```python
from build123d import *

# Parameters (mm, degrees)
SKETCH2_W           = 300
SKETCH2_H           = 200
BOSS_EXTRUDE1_DEPTH = 15
SKETCH3_W           = 240
SKETCH3_H           = 140
BOSS_EXTRUDE2_DEPTH = 15
SKETCH4_W           = 180
SKETCH4_H           = 80
BOSS_EXTRUDE3_DEPTH = 15
FILLET1_R           = 30
FILLET2_R           = 30
FILLET3_R           = 30
SCALE2_SCALE        = 2.5


with BuildPart() as part:
    # Sketch2 → Boss-Extrude1 (new body)
    with BuildSketch(Plane.XY):
        Rectangle(SKETCH2_W, SKETCH2_H)
    extrude(amount=BOSS_EXTRUDE1_DEPTH)

    # Sketch3 → Boss-Extrude2 (add)
    with BuildSketch(Plane.XY.offset(15)):
        Rectangle(SKETCH3_W, SKETCH3_H)
    extrude(amount=BOSS_EXTRUDE2_DEPTH)

    # Sketch4 → Boss-Extrude3 (add)
    with BuildSketch(Plane.XY.offset(30)):
        Rectangle(SKETCH4_W, SKETCH4_H)
    extrude(amount=BOSS_EXTRUDE3_DEPTH)

    # Fillet1
    fillet1_edges = [part.edges().sort_by_distance(p)[0] for p in [
        (-90, 40, 37.5),
        (-90, -40, 37.5),
        (90, -40, 37.5),
        (90, 40, 37.5),
    ]]
    fillet(fillet1_edges, radius=FILLET1_R)

    # Fillet2
    fillet2_edges = [part.edges().sort_by_distance(p)[0] for p in [
        (-120, 70, 22.5),
        (-120, -70, 22.5),
        (120, -70, 22.5),
        (120, 70, 22.5),
    ]]
    fillet(fillet2_edges, radius=FILLET2_R)

    # Fillet3
    fillet3_edges = [part.edges().sort_by_distance(p)[0] for p in [
        (150, -100, 7.5),
        (-150, -100, 7.5),
        (-150, 100, 7.5),
        (150, 100, 7.5),
    ]]
    fillet(fillet3_edges, radius=FILLET3_R)


with BuildPart() as part_1:
    # Scale2: scaled about (0, 0, 16.027771453)
    add(part.part.scale(SCALE2_SCALE).moved(Location((0, 0, -24.041657179))))


solid = part_1.part
```
Design review of the part built by this model. Coordinates are the model's own, in mm. A direction names the side the tool comes from. Coordinates: 2 decimals unless noted, no trailing zeros. Write each loop counter-clockwise with the first axis right and the second up, starting at its lowest first coordinate (ties: lowest second). Pieces come first, ordered by that corner, then holes. Notation, with made-up numbers: M 22.25,69 L 59.25,69 A17 ccw 59.25,86 Z; hole C -0.5,88.5 d9. An arc over 180 degrees is marked long. Answer as a JSON object with one key per item and string values.
Item 1: Add section B-B, the plane x = -123.5. Give the boundary of the cut face in (y, z).
Outcome:
{"outline": "M -250,-24.04 L 250,-24.04 L 250,13.46 L 175,13.46 L 175,50.96 L 100,50.96 L 100,88.46 L -100,88.46 L -100,50.96 L -175,50.96 L -175,13.46 L -250,13.46 Z"}
Item 2: Wall thickness on probe 1 along Z at (x, y) = (-156, 202); probe 2 along Y at (x, z) = (-29, 80); probe 3 along Z at (x, y) = (-87, -164.5): over which ranges is each line inside the solid? List them lowest first.
Outcome:
{"probe 1": "-24.04 to 13.46", "probe 2": "-100 to 100", "probe 3": "-24.04 to 50.96"}
Item 3: Machinability: for faces 3 (the flat face through (-3, 175, 32)), 4 (the cylindrical face through (203.61, 77.45, 69.97)), 5 (the cylindrical face through (-202.45, -78.61, 69.97)), 6 (the flat face through (225, 0, 69)), which of the approach directions +Z, -Z, +X, -X, +Y, -Y give a long, thin tool a straight path to every point of the face, cutting with its end or side? Answer none if there is none.
Outcome:
{"face 3": "+Z, +X, -X, +Y", "face 4": "+Z, +X, +Y", "face 5": "+Z, -X, -Y", "face 6": "+Z, +X, +Y, -Y"}
Item 4: Add section C-C, the plane y = -117. Give the boundary of the cut face in (x, z), and give its area (3 significant figures).
Outcome:
{"outline": "M -375,-24.04 L 375,-24.04 L 375,13.46 L 298.05,13.46 L 298.05,50.96 L -298.05,50.96 L -298.05,13.46 L -375,13.46 Z", "area": "50,500 mm²"}
Item 5: Add section D-D, the plane y = -49.5. Give the boundary of the cut face in (x, z), and give its area (3 significant figures).
Outcome:
{"outline": "M -375,-24.04 L 375,-24.04 L 375,13.46 L 300,13.46 L 300,50.96 L 220.89,50.96 L 220.89,88.46 L -220.89,88.46 L -220.89,50.96 L -300,50.96 L -300,13.46 L -375,13.46 Z", "area": "67,200 mm²"}
Item 6: Add section A-A, the plane z = 65.5. Give the boundary of the cut face in (x, y).
Outcome:
{"outline": "M -225,-25 A75 ccw -150,-100 L 150,-100 A75 ccw 225,-25 L 225,25 A75 ccw 150,100 L -150,100 A75 ccw -225,25 Z"}
Item 7: Insertion check: pin 1 Ø1 at (x, y) = (262.5, -26.5) entering from +Z; pin 2 Ø3 at (x, z) = (87, 23) entering from +Y; pin 3 Ø2 at (x, z) = (-199, 19.5) entering from -Y. Each pin has a flat end and moves straight along its axis. Give the tip position at first contact, or say it passes through.
Outcome:
{"pin 1": "z = 50.96", "pin 2": "y = 175", "pin 3": "y = -175"}
Item 8: Draft analysis for pull direction Z (two halves, no side actions). For faces 1 (the flat face through (-5, 226, 13.458)), 2 (the flat face through (-4, 250, -6)), state which applies: pulls with the +Z half, pulls with the -Z half, needs draft (parallel to the pull), parting line crosses it, or undercut.
Outcome:
{"face 1": "pulls with the +Z half", "face 2": "needs draft"}
